Model file for the job. Use its own axes, mm. Face numbers are marked on the shaded views. A direction names the side the tool comes from. Give positions to 0.01 mm unless a question says otherwise; leave off trailing zeros. Loops run counter-clockwise (first coordinate to the right, second up) from the corner with the lowest first, then second, coordinate; pieces in that order, holes last. Notation, with made-up numbers: (51.5, 74.5) - (65.5, 74.5) arc R16 cw to (65.5, 91.5) - close; hole circle Ø10 at (28, 64). An arc over 180 degrees is marked (long way). Use a Markdown table: item, result.
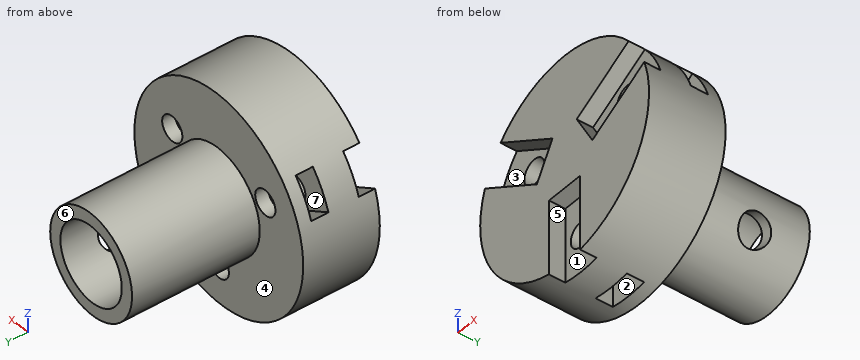
from build123d import *

# Parameters (mm, degrees)
CROQUIS1_R              = 16.5
SALIENTE_EXTRUIR1_DEPTH = 12
CROQUIS2_R              = 1.975
CROQUIS2_W              = 6.1
CROQUIS2_H              = 12
CORTAR_EXTRUIR1_DEPTH   = 2.55
CROQUIS2_2_R            = 1.975
CORTAR_EXTRUIR2_DEPTH   = 13
CROQUIS3_W              = 6.1
CROQUIS3_H              = 12
CROQUIS3_R              = 1.975
CORTAR_EXTRUIR3_DEPTH   = 2.7
CROQUIS4_R              = 8
CROQUIS4_R_2            = 6
EXTRUIR_L_MINA1_DEPTH   = 20
CORTAR_EXTRUIR4_REACH   = 31.927
CROQUIS5_R              = 2.45


with BuildPart() as part:
    # Croquis1 → Saliente-Extruir1 (new body)
    with BuildSketch(Plane(origin=(0, 0, 0), x_dir=(1, 0, 0), z_dir=(0, 1, 0))):
        Circle(CROQUIS1_R)
    extrude(amount=SALIENTE_EXTRUIR1_DEPTH)

    # Croquis2 → Cortar-Extruir1 (cut)
    with BuildSketch(Plane.XZ):
        Polygon((-12.764419162, 10.891377482), (-15.814419162, 5.608622518), (-5.422114317, -0.391377482), (-2.372114317, 4.891377482), align=None)
        with Locations((-9.09326674, 5.25)):
            Circle(CROQUIS2_R, mode=Mode.SUBTRACT)
        with Locations((0, -10.5)):
            Rectangle(CROQUIS2_W, CROQUIS2_H)
        with Locations((0, -10.5)):
            Circle(CROQUIS2_R, mode=Mode.SUBTRACT)
        Polygon((15.814419162, 5.608622518), (12.764419162, 10.891377482), (2.372114317, 4.891377482), (5.422114317, -0.391377482), align=None)
        with Locations((9.09326674, 5.25)):
            Circle(CROQUIS2_R, mode=Mode.SUBTRACT)
    extrude(amount=-CORTAR_EXTRUIR1_DEPTH, mode=Mode.SUBTRACT)

    # Croquis2_2 → Cortar-Extruir2 (cut, through all)
    with BuildSketch(Plane.XZ):
        with Locations((0, -10.5)):
            Circle(CROQUIS2_2_R)
        with Locations((-9.09326674, 5.25)):
            Circle(CROQUIS2_2_R)
        with Locations((9.09326674, 5.25)):
            Circle(CROQUIS2_2_R)
    extrude(amount=-CORTAR_EXTRUIR2_DEPTH, mode=Mode.SUBTRACT)

    # Croquis3 → Cortar-Extruir3 (cut)
    with BuildSketch(Plane(origin=(0, 10, 0), x_dir=(1, 0, 0), z_dir=(0, 1, 0))):
        with Locations((0, 10.5)):
            Rectangle(CROQUIS3_W, CROQUIS3_H)
        with Locations((0, 10.5)):
            Circle(CROQUIS3_R, mode=Mode.SUBTRACT)
        Polygon((12.764419162, -10.891377482), (15.814419162, -5.608622518), (5.422114317, 0.391377482), (2.372114317, -4.891377482), align=None)
        with Locations((9.09326674, -5.25)):
            Circle(CROQUIS3_R, mode=Mode.SUBTRACT)
        Polygon((-15.814419162, -5.608622518), (-12.764419162, -10.891377482), (-2.372114317, -4.891377482), (-5.422114317, 0.391377482), align=None)
        with Locations((-9.09326674, -5.25)):
            Circle(CROQUIS3_R, mode=Mode.SUBTRACT)
    extrude(amount=-CORTAR_EXTRUIR3_DEPTH, mode=Mode.SUBTRACT)

    # Croquis4 → Extruir-L_mina1 (add)
    with BuildSketch(Plane(origin=(0, 12, 0), x_dir=(1, 0, 0), z_dir=(0, 1, 0))):
        Circle(CROQUIS4_R)
        Circle(CROQUIS4_R_2, mode=Mode.SUBTRACT)
    extrude(amount=EXTRUIR_L_MINA1_DEPTH)

    # Croquis5 → Cortar-Extruir4 (cut, up to next)
    with BuildSketch(Plane(origin=(7.250462296, 0, -3.380946094), x_dir=(0, -1, 0), z_dir=(0.906307787, 0, -0.422618262)), mode=Mode.PRIVATE) as cortar_extruir4_sk1:
        with Locations((-24, 0)):
            Circle(CROQUIS5_R)
    cortar_extruir4_tool1 = extrude(cortar_extruir4_sk1.sketch, amount=-CORTAR_EXTRUIR4_REACH, mode=Mode.PRIVATE) & part.part
    add(cortar_extruir4_tool1.solids().sort_by_distance((7.250462, 24, -3.380946))[0], mode=Mode.SUBTRACT)


solid = part.part
(1) Slice it at B-B, the plane y = 8.5. Write the cut outline in (x, z).
Computed:
| item | result |
|---|---|
| outline | (-15.57, 5.47) arc R16.5 ccw to (-3.05, -16.22) - (-3.05, -4.5) - (3.05, -4.5) - (3.05, -16.22) arc R16.5 ccw to (15.57, 5.47) - (5.42, -0.39) - (2.37, 4.89) - (12.52, 10.75) arc R16.5 ccw to (-12.52, 10.75) - (-2.37, 4.89) - (-5.42, -0.39) - close |
(2) Mould opens along Y. For the marked faces 5, 6 and 7 say: pulls with the +Y half, pulls with the -Y half, needs draft (parallel to the pull), parting line crosses it, or undercut.
Computed:
| item | result |
|---|---|
| face 5 | needs draft |
| face 6 | pulls with the +Y half |
| face 7 | undercut |
(3) Pin check, flat tips, straight feed: P1, Ø0.8, axis at y = 9, z = -9, coming from the -X side; P2, Ø1, axis at x = -12.5, y = 11, coming from the +Z side; P3, Ø0.8, axis at x = 1, y = 9, coming from the -Z side. Stop position of each tip, or through.
Computed:
| item | result |
|---|---|
| P1 | x = -14.08 |
| P2 | z = 11.32 |
| P3 | z = -4.5 |
(4) Slice it at D-D, the plane x = -4. Write the cut outline in (y, z).
Computed:
| item | result |
|---|---|
| outline | (0, -16.01) - (12, -16.01) - (12, -6.93) - (32, -6.93) - (32, -4.47) - (12, -4.47) - (12, 4.47) - (32, 4.47) - (32, 6.93) - (12, 6.93) - (12, 16.01) - (0, 16.01) - (0, 5.83) - (2.55, 5.83) - (2.55, 2.07) - (0, 2.07) - close; hole (7.3, 2.07) - (10, 2.07) - (10, 5.83) - (7.3, 5.83) - close |
(5) Slice it at C-C, the plane z = -10.5. Write the cut outline in (x, y) (3 decimals), plus the area to 3 significant figures.
Computed:
| item | result |
|---|---|
| outline | (-12.728, 0) - (-3.05, 0) - (-3.05, 2.55) - (-1.975, 2.55) - (-1.975, 7.3) - (-3.05, 7.3) - (-3.05, 10) - (-1.975, 10) - (-1.975, 12) - (-12.728, 12) - close; (1.975, 2.55) - (3.05, 2.55) - (3.05, 0) - (12.728, 0) - (12.728, 12) - (1.975, 12) - (1.975, 10) - (3.05, 10) - (3.05, 7.3) - (1.975, 7.3) - close |
| area | 247 mm² |
(6) Drill centre lines: probe 1 along Y at (x, z) = (3, -7.5); probe 2 along Z at (x, y) = (0, 10.6) (3 decimals); probe 3 along X at (y, z) = (17, 0). Where is each one in solid material? Low to high. Write a range as [from, to].
Computed:
| item | result |
|---|---|
| probe 1 | [2.55, 7.3], [10, 12] |
| probe 2 | [-16.5, -12.475], [-8.525, 16.5] |
| probe 3 | [-8, -6], [6, 8] |
(7) 3-axis set-ups, long thin cutter, end or side, ignore diameter. For the marked faces 1, 2, 3 and 4: which of +Z, -Z, +X, -X, +Y, -Y reach the whole face in a straight line?
Computed:
| item | result |
|---|---|
| face 1 | -Z, -Y |
| face 2 | -Z |
| face 3 | -Y |
| face 4 | +Y |
(8) Slice it at A-A, the plane x = 0. Write the cut outline in (y, z) (3 decimals), plus the area to 3 significant figures.
Computed:
| item | result |
|---|---|
| outline | (0, -4.5) - (2.55, -4.5) - (2.55, -8.525) - (7.3, -8.525) - (7.3, -4.5) - (10, -4.5) - (10, -8.525) - (12, -8.525) - (12, -8) - (32, -8) - (32, -6) - (12, -6) - (12, 6) - (32, 6) - (32, 8) - (12, 8) - (12, 16.5) - (0, 16.5) - close; (2.55, -16.5) - (7.3, -16.5) - (7.3, -12.475) - (2.55, -12.475) - close; (10, -16.5) - (12, -16.5) - (12, -12.475) - (10, -12.475) - close |
| area | 386 mm² |
